Part model, mm, in its own coordinate system. Give positions to 0.01 mm unless a question says otherwise; leave off trailing zeros. Order: outer loops, then holes, each group sorted by start corner. A loop starts at its lowest first (then second) coordinate and runs counter-clockwise, first axis right, second up. Notation, with made-up numbers: (-21, 52) - (-11, 52) arc R9 ccw to (-11, 63) - close; hole circle Ø10 at (-8.5, 69). An arc over 180 degrees is marked (long way). One line per item, written item: value.
```python
from build123d import *

# Parameters (mm, degrees)
SKETCH1_R                   = 25.4
BOSS_EXTRUDE1_DEPTH         = 127
F_1_4_20_TAPPED_HOLE1_D     = 5.1054
F_1_4_20_TAPPED_HOLE1_DEPTH = 25.4
F_1_4_20_TAPPED_HOLE1_TIP   = 1.533816902


with BuildPart() as part:
    # Sketch1 → Boss-Extrude1 (new body)
    with BuildSketch(Plane(origin=(0, 0, 0), x_dir=(1, 0, 0), z_dir=(0, 1, 0))):
        Circle(SKETCH1_R)
    extrude(amount=BOSS_EXTRUDE1_DEPTH)

    # 1/4-20 Tapped Hole1
    with Locations(Plane(origin=(0, 0, 0), x_dir=(-1, 0, 0), z_dir=(0, -1, 0))):
        with Locations((12.7, 0), (-12.7, 0)):
            Hole(F_1_4_20_TAPPED_HOLE1_D / 2, depth=F_1_4_20_TAPPED_HOLE1_DEPTH)
            with Locations((0, 0, -(F_1_4_20_TAPPED_HOLE1_DEPTH + F_1_4_20_TAPPED_HOLE1_TIP / 2))):  # 118° drill point
                Cone(0, F_1_4_20_TAPPED_HOLE1_D / 2, F_1_4_20_TAPPED_HOLE1_TIP, mode=Mode.SUBTRACT)


solid = part.part
```
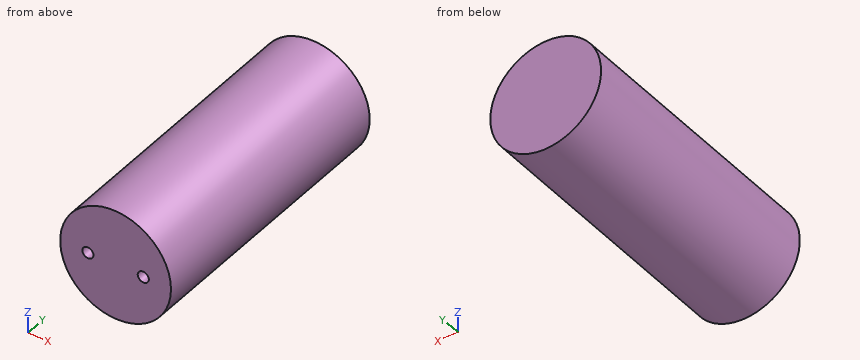
1) Cut at B-B, the plane x = 22. Give the cut face in (y, z).
Outcome:
outline: (0, -12.69) - (127, -12.69) - (127, 12.69) - (0, 12.69) - close
2) Pin check, flat tips, straight feed: pin 1 (8 mm diameter, centred on x = 14.5, y = 70, fed in from +Z); pin 2 (2 mm diameter, centred on x = -6, y = 56, fed in from -Z); pin 3 (2 mm diameter, centred on x = -17.5, y = 76.5, fed in from -Z). Stop position of each tip, or through.
Outcome:
pin 1: stops at z = 23.13
pin 2: stops at z = -24.9
pin 3: stops at z = -19.31
3) Cut at C-C, the plane z = -7. Give the cut face in (x, y), then the cut area to 3 significant figures.
Outcome:
outline: (-24.42, 0) - (24.42, 0) - (24.42, 127) - (-24.42, 127) - close
area: 6,200 mm^2
4) Cut at A-A, the plane y = 64.5. Give the cut face in (x, z).
Outcome:
outline: circle Ø50.8 at (0, 0)
5) Drill centre lines: line 1 along Z through (x, y) = (-12.7, 5.75); line 2 along Z through (x, y) = (1, 21); line 3 along Z through (x, y) = (12, 19). Where is each one in solid material? Low to high. Write a range as from..to.
Outcome:
line 1: z = -22..-2.55, 2.55..22
line 2: z = -25.38..25.38
line 3: z = -22.39..-2.45, 2.45..22.39
